Check sheet for the drawn part. Datum: minimum x, y, z corner. Units: mm. Give positions to 0.01 mm unless a question says otherwise; leave off trailing zeros. Order: outer loops, then holes, each group sorted by start corner. A loop starts at its lowest first (then second) coordinate and runs counter-clockwise, first axis right, second up. Notation, with made-up numbers: (77.5, 32.5) -> (87.5, 32.5) arc R10 ccw to (87.5, 47.5) -> close; hole circle Ø7 at (-23.5, 53.25). An arc over 180 degrees is marked (long way). Answer in a Markdown table with one row per item. Add a question column.
(1) Go/stop test with a flat-tipped pin: pin 1 (2 mm diameter, centred on x = 4.5, z = 3, fed in from +Y). Record where the tip stops, or that it passes through.
(2) Cross-section at A-A (z = 2.85). Record the cut outline in (x, y), then the cut area to 3 significant figures.
(3) Release check for a two-part mould opening along Y. For the marked faces 1, 2 and 3 record: released by +Y, released by -Y, zero draft, split by the parting line, or undercut.
(4) Thickness scan on L1, parallel to X at y = 6.25, z = 2.7 (1 decimal); L2, parallel to X at y = 3.75, z = 1.65 (1 decimal); L3, parallel to Y at x = 2.75, z = 3.4 (1 decimal). Record the ranges inside material, lowest first. Write a range as [from, to].
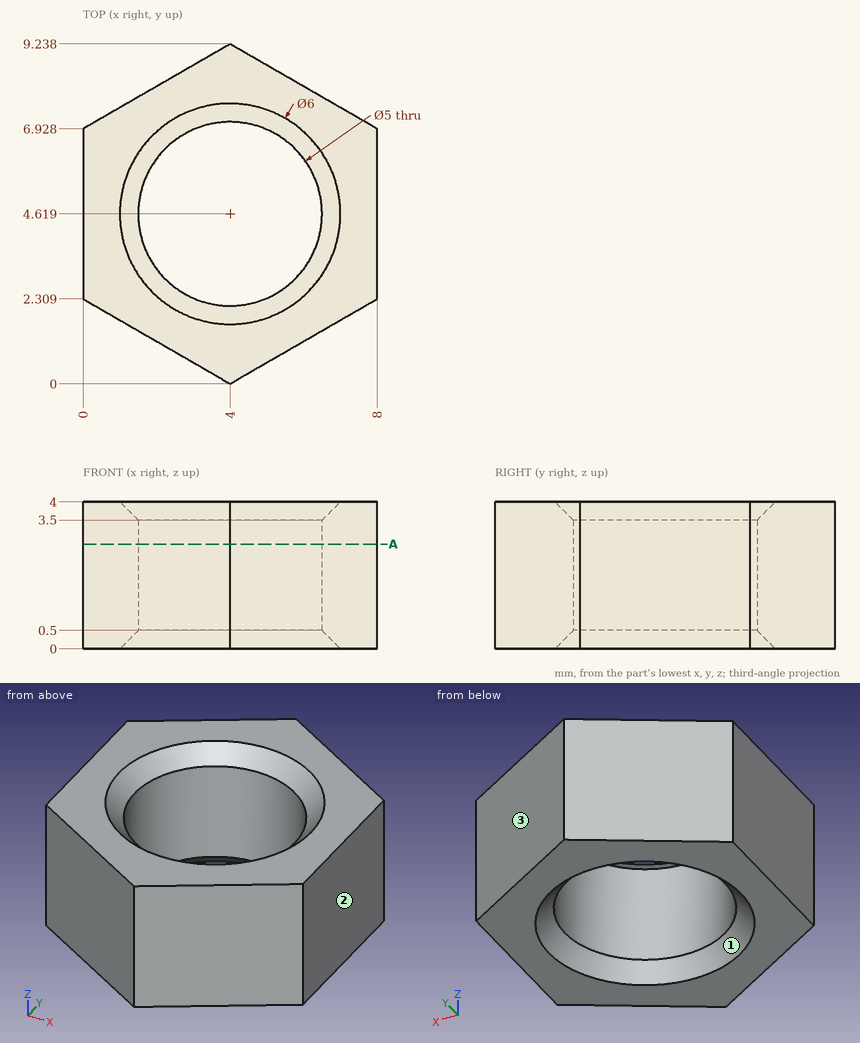
Answer below:
| question | item | result |
|---|---|---|
| 1 | pin 1 | stops at y = 9.24 |
| 2 | outline | (0, 2.31) -> (4, 0) -> (8, 2.31) -> (8, 6.93) -> (4, 9.24) -> (0, 6.93) -> close; hole circle Ø5 at (4, 4.62) |
| 2 | area | 35.8 mm² |
| 3 | face 1 | undercut |
| 3 | face 2 | zero draft |
| 3 | face 3 | released by +Y |
| 4 | L1 | x = [0, 2.1], [5.9, 8] |
| 4 | L2 | x = [0, 1.7], [6.3, 8] |
| 4 | L3 | y = [0.7, 2.5], [6.8, 8.5] |
